Geometry: final body of the model. Coordinates: model frame, mm. A direction names the side the tool comes from. Coordinates: 2 decimals unless noted, no trailing zeros. Order: outer loops, then holes, each group sorted by start corner. A loop starts at its lowest first (then second) coordinate and runs counter-clockwise, first axis right, second up. Notation, with made-up numbers: (51.25, 81.5) -> (94.25, 81.5) arc R10 cw to (94.25, 85.5) -> close; hole circle Ø1 at (84.5, 19). An arc over 180 degrees is marked (long way). Answer in a Markdown table with one row per item. Add a question column.
1) Section query A-A on y = 0. Return the cut outline in (x, z).
2) Ray query, line 1 (Y direction, x = 0, z = 8.4); line 2 (Y direction, x = 0, z = 9.5); line 3 (X direction, y = -14, z = 7.75). Return the intervals inside material, ascending. Write a range as from..to.
3) Set-up query: faces 1 (the face through (11, -4, 11)), 2 (the face through (-1.5, 11.4, 10)), 3 (the face through (-15.5, 0, 4)). Return all of +Z, -Z, +X, -X, +Y, -Y with unobstructed straight access to the full face (end or side cutting, diameter ignored); none if empty.
4) Section query B-B on x = 0. Return the cut outline in (y, z), then the cut area to 3 significant figures.
5) Section query C-C on x = -14.5. Return the cut outline in (y, z).
6) Section query D-D on z = 10.5. Return the cut outline in (x, y), then the cut area to 3 significant figures.
7) Contact query for flat-ended pins moving along their axis: P1, Ø7, axis at x = 0, y = -2, coming from the +Z side; P2, Ø5, axis at x = -11.5, z = 3.5, coming from the +Y side; P3, Ø3.5, axis at y = -2.5, z = 2, coming from the +X side. Output: stop coordinate, or through.
```python
from build123d import *

# Parameters (mm, degrees)
F0_R      = 18
F0_R_2    = 16.75
F0_R_3    = 12.5
F0_R_4    = 11.5
F1_DEPTH  = 10
F2_R      = 16.75
F3_DEPTH  = 3
F4_R      = 12.5
F5_DEPTH  = 4
F6_R      = 11.5
F7_DEPTH  = 2
F9_R      = 8
F10_DEPTH = 33.5


# Not quite as in the source:
# - the program builds the solid bodies; features that only make, move or delete a surface that nothing else refers to are left out


with BuildPart() as f1:
    # F0 (on Top) → F1 (new body)
    with BuildSketch(Plane.XY):
        Circle(F0_R)
        Circle(F0_R_2, mode=Mode.SUBTRACT)
        Circle(F0_R_2)
        Circle(F0_R_3, mode=Mode.SUBTRACT)
        Circle(F0_R_3)
        Circle(F0_R_4, mode=Mode.SUBTRACT)
        Circle(F0_R_4)
    extrude(amount=F1_DEPTH)

    # F2 (on face) → F3 (cut)
    with BuildSketch(Plane.XY.offset(10)):
        Circle(F2_R)
    extrude(amount=-F3_DEPTH, mode=Mode.SUBTRACT)

    # F4 (on face) → F5 (join)
    with BuildSketch(Plane.XY.offset(7)):
        Circle(F4_R)
    extrude(amount=F5_DEPTH)

    # F6 (on face) → F7 (cut)
    with BuildSketch(Plane.XY.offset(11)):
        Circle(F6_R)
    extrude(amount=-F7_DEPTH, mode=Mode.SUBTRACT)

    # F9 (on offset) → F10 (cut)
    with BuildSketch(Plane.YZ.offset(18)):
        Circle(F9_R)
    extrude(amount=-F10_DEPTH, mode=Mode.SUBTRACT)


solid = f1.part
```
Result:
| question | item | result |
|---|---|---|
| 1 | outline | (-18, 0) -> (-15.5, 0) -> (-15.5, 7) -> (-16.75, 7) -> (-16.75, 10) -> (-18, 10) -> close; (-12.5, 8) -> (12.5, 8) -> (12.5, 11) -> (11.5, 11) -> (11.5, 9) -> (-11.5, 9) -> (-11.5, 11) -> (-12.5, 11) -> close; (16.75, 8) -> (18, 8) -> (18, 10) -> (16.75, 10) -> close |
| 2 | line 1 | -18..-16.75, -12.5..12.5, 16.75..18 |
| 2 | line 2 | -18..-16.75, -12.5..-11.5, 11.5..12.5, 16.75..18 |
| 2 | line 3 | -11.31..-9.2, 9.2..11.31 |
| 3 | face 1 | +Z, +X, -X, +Y, -Y |
| 3 | face 2 | +Z |
| 3 | face 3 | -Z, +X |
| 4 | outline | (-18, 0) -> (-8, 0) arc R8 cw to (8, 0) -> (18, 0) -> (18, 10) -> (16.75, 10) -> (16.75, 7) -> (12.5, 7) -> (12.5, 11) -> (11.5, 11) -> (11.5, 9) -> (-11.5, 9) -> (-11.5, 11) -> (-12.5, 11) -> (-12.5, 7) -> (-16.75, 7) -> (-16.75, 10) -> (-18, 10) -> close |
| 4 | area | 213 mm2 |
| 5 | outline | (-10.67, 0) -> (-8, 0) arc R8 cw to (-3.87, 7) -> (-8.39, 7) -> (-8.39, 10) -> (-10.67, 10) -> close; (3.87, 7) arc R8 cw to (8, 0) -> (10.67, 0) -> (10.67, 10) -> (8.39, 10) -> (8.39, 7) -> close |
| 6 | outline | circle Ø25 at (0, 0); hole circle Ø23 at (0, 0) |
| 6 | area | 75.4 mm2 |
| 7 | P1 | z = 9 |
| 7 | P2 | y = 15.59 |
| 7 | P3 | x = -15.5 |
